Verification items for this drawing (mm, ordinates from the low corner). A direction names the side the tool comes from. Give positions to 0.01 mm unless a question says otherwise; leave off trailing zeros. Loops run counter-clockwise (first coordinate to the right, second up) from the corner with the lowest first, then second, coordinate; pieces in that order, holes last. Notation, with made-up numbers: (6, 6.5) -> (23, 6.5) arc R16 ccw to (23, 18.5) -> close; hole circle Ø5 at (-9.5, 79.25). An arc over 180 degrees is marked (long way). Write item = value, one per line.
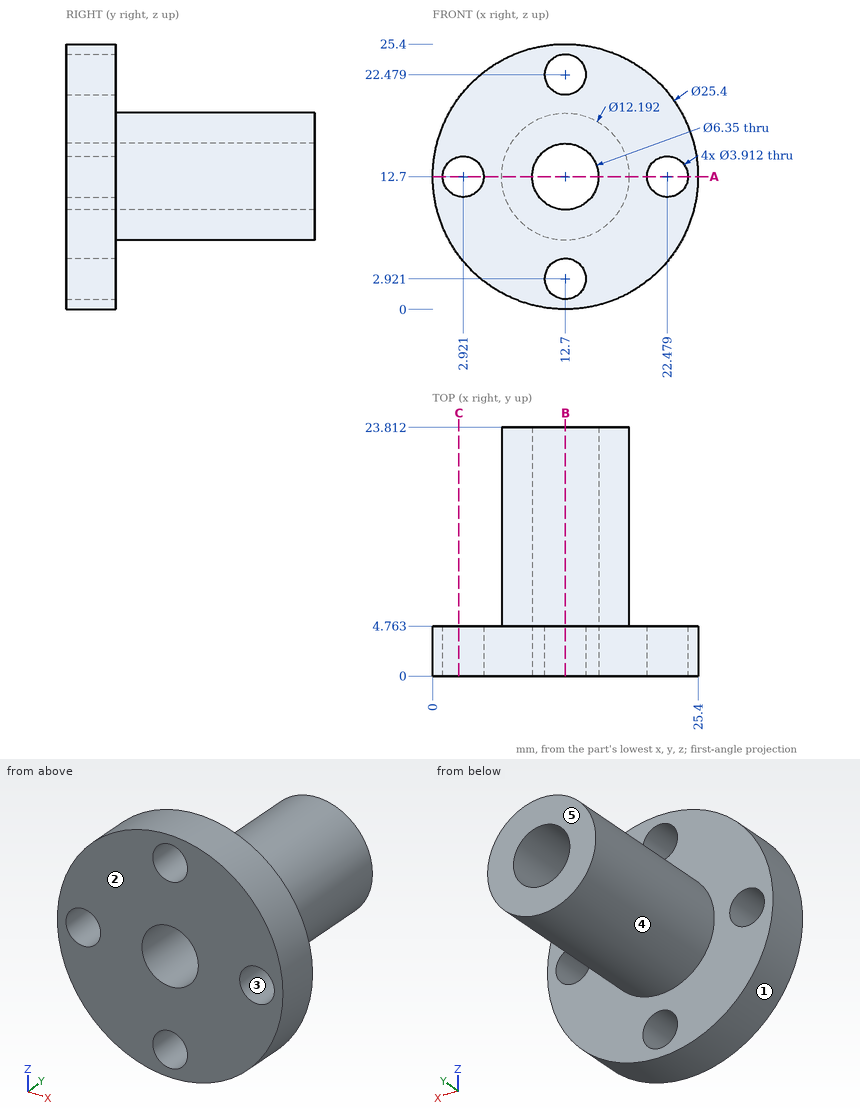
Item 1: Section check C-C, the plane x = 2.5. Record the cut outline in (y, z).
Answer:
outline = (0, 5.13) -> (4.76, 5.13) -> (4.76, 10.79) -> (0, 10.79) -> close; (0, 14.61) -> (4.76, 14.61) -> (4.76, 20.27) -> (0, 20.27) -> close
Item 2: Tool access check on the marked faces 4 and 5. Record the directions out of +Z, -Z, +X, -X, +Y, -Y that give a thin tool (end or side, any length) a straight path to the whole face; none if there is none.
Answer:
face_4 = +Y
face_5 = +Z, -Z, +X, -X, +Y
Item 3: Section check A-A, the plane z = 12.7. Record the cut outline in (x, y) (1 decimal), plus the area to 3 significant figures.
Answer:
outline = (0, 0) -> (1, 0) -> (1, 4.8) -> (0, 4.8) -> close; (4.9, 0) -> (9.5, 0) -> (9.5, 23.8) -> (6.6, 23.8) -> (6.6, 4.8) -> (4.9, 4.8) -> close; (15.9, 0) -> (20.5, 0) -> (20.5, 4.8) -> (18.8, 4.8) -> (18.8, 23.8) -> (15.9, 23.8) -> close; (24.4, 0) -> (25.4, 0) -> (25.4, 4.8) -> (24.4, 4.8) -> close
area = 165 mm^2
Item 4: Gauge pin test, flat ends, axial feed: pin 1 (10 mm diameter, centred on y = 16, z = 15.5, fed in from -X); pin 2 (2 mm diameter, centred on x = 3.5, z = 22.5, fed in from +Y); pin 3 (2 mm diameter, centred on y = 5, z = 8.5, fed in from +X). Record the tip position at first contact, or that the pin passes through.
Answer:
pin_1 = 6.6
pin_2 = 4.76
pin_3 = 24.98
Item 5: Thickness scan on L1, parallel to X at y = 1.6, z = 12.7 (1 decimal); L2, parallel to Y at x = 21.5, z = 7.75. Record the ranges inside material, lowest first. Write a range as [from, to].
Answer:
L1 = [0, 1], [4.9, 9.5], [15.9, 20.5], [24.4, 25.4]
L2 = [0, 4.76]
Item 6: Draft check along X on the marked faces 1, 2 and 3. Enter one of: +X half, -X half, draft (parallel to the pull), parting line (faces both ways), or undercut.
Answer:
face_1 = parting line
face_2 = draft
face_3 = undercut
Item 7: Section check B-B, the plane x = 12.7. Record the cut outline in (y, z) (1 decimal).
Answer:
outline = (0, 0) -> (4.8, 0) -> (4.8, 1) -> (0, 1) -> close; (0, 4.9) -> (4.8, 4.9) -> (4.8, 6.6) -> (23.8, 6.6) -> (23.8, 9.5) -> (0, 9.5) -> close; (0, 15.9) -> (23.8, 15.9) -> (23.8, 18.8) -> (4.8, 18.8) -> (4.8, 20.5) -> (0, 20.5) -> close; (0, 24.4) -> (4.8, 24.4) -> (4.8, 25.4) -> (0, 25.4) -> close
